The listing builds one solid part. Answer for the finished solid, in the listing's coordinates (mm). Round coordinates to 2 decimals unless told otherwise and drop trailing zeros. Write each loop counter-clockwise with the first axis right and the second up, starting at its lowest first coordinate (ties: lowest second). Pieces come first, ordered by that corner, then holes. Notation, with made-up numbers: M -17,-29.5 L -1,-29.5 A19 cw -1,-5.5 Z; hole C 6,-36 d10. An arc over 180 degrees is marked long. One line per item, written item: value. Start each with the question number.
(1) Section D-D (x = 24) is taken. Determine the outline of the cut face in (y, z), plus the area to 3 significant figures.
(2) Given P1, Ø1.8, axis at x = 0, z = 13.58, coming from the +Y side; P2, Ø2.5, axis at y = -1, z = 102, coming from the +X side; P3, Ø1.4, axis at y = 0, z = 107, coming from the +X side, each flat-ended and moving along its own axis, determine where each tip first touches the part or whether it passes through.
(3) Section B-B (z = 2.5) is taken. Determine the outline of the cut face in (x, y), plus the area to 3 significant figures.
(4) Consider probe 1 along Z at (x, y) = (10.85, 0.25); probe 2 along Y at (x, z) = (11.05, 97.5); probe 3 along X at (y, z) = (2.75, 13.5). Determine where each line is inside the solid, lowest interval first.
(5) Section C-C (y = 3.75) is taken. Determine the outline of the cut face in (x, z).
(6) Section A-A (x = 9.5) is taken. Determine the outline of the cut face in (y, z), plus the area to 3 significant figures.
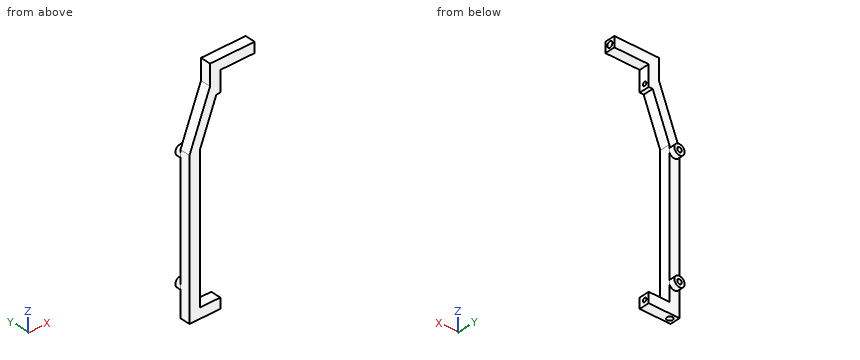
```python
from build123d import *

# Parameters (mm, degrees)
SKETCH1_W           = 5
SKETCH1_H           = 5
BOSS_EXTRUDE1_DEPTH = 74.08
SKETCH2_R           = 1.4
CUT_EXTRUDE1_DEPTH  = 10
SKETCH3_W           = 5
SKETCH3_H           = 5
BOSS_EXTRUDE2_DEPTH = 10
SKETCH4_R           = 0.95
CUT_EXTRUDE2_DEPTH  = 5
SKETCH5_R           = 2.5
SKETCH5_R_2         = 1.1
BOSS_EXTRUDE3_DEPTH = 2.8
SKETCH6_W           = 5
SKETCH6_H           = 5
SKETCH6_R           = 0.95
BOSS_EXTRUDE4_DEPTH = 5
BOSS_EXTRUDE5_DEPTH = 5
BOSS_EXTRUDE6_START = 2.5
BOSS_EXTRUDE6_DEPTH = 5
SKETCH9_R           = 1.4
CUT_EXTRUDE3_DEPTH  = 10


with BuildPart() as part:
    # Sketch1 → Boss-Extrude1 (new body)
    with BuildSketch(Plane.XY):
        Rectangle(SKETCH1_W, SKETCH1_H)
    extrude(amount=BOSS_EXTRUDE1_DEPTH)

    # Sketch2 → Cut-Extrude1 (cut)
    with BuildSketch(Plane(origin=(0, 0, 0), x_dir=(-1, 0, 0), z_dir=(0, 0, -1))):
        Circle(SKETCH2_R)
    extrude(amount=-CUT_EXTRUDE1_DEPTH, mode=Mode.SUBTRACT)

    # Sketch3 → Boss-Extrude2 (add)
    with BuildSketch(Plane(origin=(2.5, 0, 0), x_dir=(0, 0, -1), z_dir=(1, 0, 0))):
        with Locations((-2.5, 0)):
            Rectangle(SKETCH3_W, SKETCH3_H)
    extrude(amount=BOSS_EXTRUDE2_DEPTH)

    # Sketch4 → Cut-Extrude2 (cut)
    with BuildSketch(Plane(origin=(12.5, 0, 0), x_dir=(0, 0, -1), z_dir=(1, 0, 0))):
        with Locations(Location((-2.5, 0.25, 0), (0, 0, 90))):
            Circle(SKETCH4_R)
    extrude(amount=-CUT_EXTRUDE2_DEPTH, mode=Mode.SUBTRACT)

    # Sketch5 → Boss-Extrude3 (add)
    # profile 1 of 2: a face of its own
    with BuildSketch(Plane(origin=(0, 2.5, 0), x_dir=(1, 0, 0), z_dir=(0, 1, 0))):
        with Locations(Location((0, -13.58, 0), (0, 0, 180))):
            Circle(SKETCH5_R)
        with Locations(Location((0, -13.58, 0), (0, 0, 270))):
            Circle(SKETCH5_R_2, mode=Mode.SUBTRACT)
    # profile 2 of 2: a face of its own
    with BuildSketch(Plane(origin=(0, 2.5, 0), x_dir=(1, 0, 0), z_dir=(0, 1, 0))):
        with Locations(Location((0, -71.58, 0), (0, 0, 270))):
            Circle(SKETCH5_R)
        with Locations(Location((0, -71.58, 0), (0, 0, 270))):
            Circle(SKETCH5_R_2, mode=Mode.SUBTRACT)
    extrude(amount=BOSS_EXTRUDE3_DEPTH)



with BuildPart() as body_2:
    # Sketch6 → Boss-Extrude4 (new body)
    with BuildSketch(Plane(origin=(12.5, 0, 0), x_dir=(0, 0, -1), z_dir=(1, 0, 0))):
        with Locations((-97.5, 0)):
            Rectangle(SKETCH6_W, SKETCH6_H)
        with Locations(Location((-97.5, 0.25, 0), (0, 0, 90))):
            Circle(SKETCH6_R, mode=Mode.SUBTRACT)
    extrude(amount=-BOSS_EXTRUDE4_DEPTH)


with BuildPart() as part_1:
    add(part.part)

    add(body_2.part)  # Boss-Extrude5 merges body 2
    # Sketch7 → Boss-Extrude5 (add)
    with BuildSketch(Plane(origin=(0, 2.5, 0), x_dir=(1, 0, 0), z_dir=(0, 1, 0))):
        Polygon((7.5, -100), (-2.5, -74.08), (2.5, -74.08), (10.570987654, -95), (7.5, -95), align=None)
    extrude(amount=-BOSS_EXTRUDE5_DEPTH)

    # Sketch8 → Boss-Extrude6 (add)
    with BuildSketch(Plane(origin=(0, 0, 0), x_dir=(1, 0, 0), z_dir=(0, 1, 0)).offset(BOSS_EXTRUDE6_START)):
        Polygon((7.5, -100), (7.5, -110), (29.2, -110), (29.2, -105), (12.5, -105), (12.5, -100), align=None)
    extrude(amount=-BOSS_EXTRUDE6_DEPTH)

    # Sketch9 → Cut-Extrude3 (cut)
    with BuildSketch(Plane(origin=(29.2, 0, 0), x_dir=(0, 0, -1), z_dir=(1, 0, 0))):
        with Locations((-107.5, 0)):
            Circle(SKETCH9_R)
    extrude(amount=-CUT_EXTRUDE3_DEPTH, mode=Mode.SUBTRACT)


solid = part_1.part
```
Recorded:
1. outline: M -2.5,105 L 2.5,105 L 2.5,110 L -2.5,110 Z; hole C 0,107.5 d2.8
1. area: 18.8 mm2
2. P1: stops at y = 2.5
2. P2: stops at x = 12.5
2. P3: stops at x = 19.2
3. outline: M -2.5,-2.5 L 12.5,-2.5 L 12.5,-0.7 L 7.5,-0.7 L 7.5,1.2 L 12.5,1.2 L 12.5,2.5 L -2.5,2.5 Z; hole C 0,0 d2.8
3. area: 59.3 mm2
4. probe 1: z = 0 to 1.55, 3.45 to 5, 95 to 96.55, 98.45 to 110
4. probe 2: y = -2.5 to -0.7, 1.2 to 2.5
4. probe 3: x = -2.5 to -1.1, 1.1 to 2.5
5. outline: C 0,13.58 d5; C 0,71.58 d5; hole C 0,13.58 d2.2; hole C 0,71.58 d2.2
6. outline: M -2.5,0 L 2.5,0 L 2.5,5 L -2.5,5 Z; M -2.5,92.22 L 2.5,92.22 L 2.5,110 L -2.5,110 Z; hole C 0.25,2.5 d1.9; hole C 0.25,97.5 d1.9
6. area: 108 mm2
